Check sheet for the modelled part. Datum: model origin and axes. Units: mm. A direction names the side the tool comes from. Round coordinates to 2 decimals unless told otherwise and drop trailing zeros. Loops run counter-clockwise (first coordinate to the right, second up) from the corner with the lowest first, then second, coordinate; pieces in that order, holes last. Notation, with made-up numbers: (76.5, -18.75) -> (102.5, -18.75) arc R11 cw to (102.5, -14.75) -> close; hole circle Ø10 at (43, 11). An arc over 180 degrees is marked (long way). Use one line per item in the form item = value. Start each with the question number.
(1) Material ranges on probe 1 along Y at (x, z) = (1, 0); probe 2 along Z at (x, y) = (1.5, 7.25); probe 3 along Y at (x, z) = (4, 2.25), recorded low to high. Write a range as [from, to].
(2) Sectioned sample at D-D (z = -4). Record the cut outline in (x, y), and give its area (3 significant figures).
(3) Sectioned sample at C-C (x = -1). Record the cut outline in (y, z) (3 decimals), and give its area (3 significant figures).
(4) Draft check along Y on faces 1 (the cylindrical face through (0.068, 4.267, 0.688)), 2 (the flat face through (0, 12.192, 0)), 3 (the flat face through (4, 2.54, 4)), 4 (the flat face through (-4.826, 4, 0)). Enter one of: released by +Y, released by -Y, zero draft, split by the parting line, or undercut.
(5) Set-up check for faces 5 (the flat face through (0, 0, 0)), 6 (the flat face through (-4, 2.54, -4)), 7 (the flat face through (4, 2.54, -4)), 8 (the cylindrical face through (-3.83, 1.252, 2.937)), 9 (the flat face through (-4, 2.54, 4)): record each of +Z, -Z, +X, -X, +Y, -Y from which the full face is reachable in a straight line by a thin tool's end or side.
(6) Sectioned sample at A-A (z = -2.25). Record the cut outline in (x, y), and give its area (3 significant figures).
(7) Sectioned sample at B-B (y = 9.5). Record the cut outline in (x, z).
from build123d import *

# Parameters (mm, degrees)
SKETCH1_R           = 4.826
BOSS_EXTRUDE1_DEPTH = 2.54
SKETCH2_W           = 9.652
SKETCH2_H           = 9.652
BOSS_EXTRUDE2_DEPTH = 9.652
SKETCH3_R           = 3.175
CUT_EXTRUDE1_DEPTH  = 9.652


with BuildPart() as part:
    # Sketch1 → Boss-Extrude1 (new body)
    with BuildSketch(Plane(origin=(0, 0, 0), x_dir=(1, 0, 0), z_dir=(0, 1, 0))):
        Circle(SKETCH1_R)
    extrude(amount=BOSS_EXTRUDE1_DEPTH)

    # Sketch2 → Boss-Extrude2 (add)
    with BuildSketch(Plane(origin=(0, 2.54, 0), x_dir=(1, 0, 0), z_dir=(0, 1, 0))):
        Rectangle(SKETCH2_W, SKETCH2_H)
    extrude(amount=BOSS_EXTRUDE2_DEPTH)

    # Sketch3 → Cut-Extrude1 (cut)
    with BuildSketch(Plane(origin=(4.826, 0, 0), x_dir=(0, 0, -1), z_dir=(1, 0, 0))):
        with Locations((0, 7.366)):
            Circle(SKETCH3_R)
    extrude(amount=-CUT_EXTRUDE1_DEPTH, mode=Mode.SUBTRACT)


solid = part.part
Checks:
q1.probe_1 = [0, 4.19], [10.54, 12.19]
q1.probe_2 = [-4.83, -3.17], [3.17, 4.83]
q1.probe_3 = [0, 5.13], [9.61, 12.19]
q2.outline = (-4.83, 2.54) -> (-2.7, 2.54) -> (-2.7, 0) -> (2.7, 0) -> (2.7, 2.54) -> (4.83, 2.54) -> (4.83, 12.19) -> (-4.83, 12.19) -> close
q2.area = 107 mm2
q3.outline = (0, -4.721) -> (2.54, -4.721) -> (2.54, -4.826) -> (12.192, -4.826) -> (12.192, 4.826) -> (2.54, 4.826) -> (2.54, 4.721) -> (0, 4.721) -> close; hole circle Ø6.35 at (7.366, 0)
q3.area = 85.5 mm2
q4.face_1 = undercut
q4.face_2 = released by +Y
q4.face_3 = released by -Y
q4.face_4 = zero draft
q5.face_5 = +Z, -Z, +X, -X, -Y
q5.face_6 = -Z, -X, -Y
q5.face_7 = -Z, +X, -Y
q5.face_8 = -Y
q5.face_9 = +Z, -X, -Y
q6.outline = (-4.83, 2.54) -> (-4.27, 2.54) -> (-4.27, 0) -> (4.27, 0) -> (4.27, 2.54) -> (4.83, 2.54) -> (4.83, 5.13) -> (-4.83, 5.13) -> close; (-4.83, 9.61) -> (4.83, 9.61) -> (4.83, 12.19) -> (-4.83, 12.19) -> close
q6.area = 71.6 mm2
q7.outline = (-4.83, -4.83) -> (4.83, -4.83) -> (4.83, -2.35) -> (-4.83, -2.35) -> close; (-4.83, 2.35) -> (4.83, 2.35) -> (4.83, 4.83) -> (-4.83, 4.83) -> close
